Autodesk Inventor part; units mm, degrees
ref_plane "YZ Plane" through (0, 0, 0) normal (1, 0, 0) x (0, 1, 0)
ref_plane "XZ Plane" through (0, 0, 0) normal (0, 1, 0) x (-1, 0, 0)
ref_plane "XY Plane" through (0, 0, 0) normal (0, 0, 1) x (1, 0, 0)
sketch "Sketch1" plane through (0, 0, 0) normal (0, 1, 0) x (-1, 0, 0)
  line L0 (9, -10) -> (-9, -10)
  line L1 (-10, -9) -> (-10, 9)
  line L2 (-9, 10) -> (9, 10)
  line L3 (10, 9) -> (10, -9)
  line L4 (10, 10) -> (-10, -10) construction
  line L5 (10, -10) -> (-10, 10) construction
  arc A0 (10, 9) -> (9, 10) centre (9, 9) ccw
  arc A1 (9, -10) -> (10, -9) centre (9, -9) ccw
  arc A2 (-10, -9) -> (-9, -10) centre (-9, -9) ccw
  arc A3 (-9, 10) -> (-10, 9) centre (-9, 9) ccw
  point P0 (0, 0)
  point P1 (0, 0)
  dimension "d7" = 20
  dimension "d9" = 20
  dimension "d10" = 1
extrude "Extrusion1" add sketch "Sketch1" along normal blind 5
sketch "Sketch2" plane through (0, 5, 0) normal (0, 1, 0) x (1, 0, 0)
  line L0 (-10, 9) -> (-10, -9)
  arc A0 (-10, -9) -> (-9, -10) centre (-9, -9) ccw
  line L1 (-9, -10) -> (9, -10)
  arc A1 (9, -10) -> (10, -9) centre (9, -9) ccw
  line L2 (10, -9) -> (10, 9)
  arc A2 (10, 9) -> (9, 10) centre (9, 9) ccw
  line L3 (9, 10) -> (-9, 10)
  arc A3 (-9, 10) -> (-10, 9) centre (-9, 9) ccw
  line L4 (9, -11.5) -> (-9, -11.5)
  arc A4 (-11.5, -9) -> (-9, -11.5) centre (-9, -9) ccw
  line L5 (-11.5, -9) -> (-11.5, 9)
  arc A5 (-9, 11.5) -> (-11.5, 9) centre (-9, 9) ccw
  line L6 (-9, 11.5) -> (9, 11.5)
  arc A6 (11.5, 9) -> (9, 11.5) centre (9, 9) ccw
  line L7 (11.5, 9) -> (11.5, -9)
  arc A7 (9, -11.5) -> (11.5, -9) centre (9, -9) ccw
  circle A8 centre (0, 0) radius 2.75
  dimension "d16" = 1.5
  dimension "d19" = 5.5
extrude "Extrusion3" add sketch "Sketch2" along normal blind 1 contours A3 L3 A2 L2 A1 L1 A0 L0 | L4 A4 L5 A5 L6 A6 L7 A7
sketch "Sketch3" plane through (0, 0, 0) normal (0, -1, 0) x (1, 0, 0)
  circle A0 centre (0, 0) radius 4
  arc A1 (-6, -1) -> (-6, 1) centre (-6, 0) ccw
  arc A2 (-8, 1) -> (-8, -1) centre (-8, 0) ccw
  line L0 (-6, -1) -> (-8, -1)
  line L1 (-6, 1) -> (-8, 1)
  line L2 (0, 0) -> (-5, 0) construction
  arc A3 (-3.5355, -4.9497) -> (-4.9497, -3.5355) centre (-4.2426, -4.2426) ccw
  line L3 (-3.5355, -4.9497) -> (-4.9497, -6.364)
  line L4 (-4.9497, -3.5355) -> (-6.364, -4.9497)
  arc A4 (-6.364, -4.9497) -> (-4.9497, -6.364) centre (-5.6569, -5.6569) ccw
  arc A5 (1, -6) -> (-1, -6) centre (0, -6) ccw
  line L5 (1, -6) -> (1, -8)
  line L6 (-1, -6) -> (-1, -8)
  arc A6 (-1, -8) -> (1, -8) centre (0, -8) ccw
  arc A7 (4.9497, -3.5355) -> (3.5355, -4.9497) centre (4.2426, -4.2426) ccw
  line L7 (4.9497, -3.5355) -> (6.364, -4.9497)
  line L8 (3.5355, -4.9497) -> (4.9497, -6.364)
  arc A8 (4.9497, -6.364) -> (6.364, -4.9497) centre (5.6569, -5.6569) ccw
  arc A9 (6, 1) -> (6, -1) centre (6, 0) ccw
  line L9 (6, 1) -> (8, 1)
  line L10 (6, -1) -> (8, -1)
  arc A10 (8, -1) -> (8, 1) centre (8, 0) ccw
  arc A11 (3.5355, 4.9497) -> (4.9497, 3.5355) centre (4.2426, 4.2426) ccw
  line L11 (3.5355, 4.9497) -> (4.9497, 6.364)
  line L12 (4.9497, 3.5355) -> (6.364, 4.9497)
  arc A12 (6.364, 4.9497) -> (4.9497, 6.364) centre (5.6569, 5.6569) ccw
  arc A13 (-1, 6) -> (1, 6) centre (0, 6) ccw
  line L13 (-1, 6) -> (-1, 8)
  line L14 (1, 6) -> (1, 8)
  arc A14 (1, 8) -> (-1, 8) centre (0, 8) ccw
  arc A15 (-4.9497, 3.5355) -> (-3.5355, 4.9497) centre (-4.2426, 4.2426) ccw
  line L15 (-4.9497, 3.5355) -> (-6.364, 4.9497)
  line L16 (-3.5355, 4.9497) -> (-4.9497, 6.364)
  arc A16 (-4.9497, 6.364) -> (-6.364, 4.9497) centre (-5.6569, 5.6569) ccw
  dimension "d24" = 2
  dimension "d25" = 2
  dimension "d26" = 2
  dimension "d27" = 6
  dimension "d28" = 360
  dimension "d29" = 16
  dimension "d37" = 8
extrude "Extrusion4" cut sketch "Sketch3" against normal blind 1
hole "Hole1" at (0, 5, 0) direction (0, -1, 0) diameter 5.5 depth 3
equation "\"d7\" = button_side"
equation "\"d9\" = d7"
equation "\"d24\" = d25"
equation "\"d25\" = d26"
equation "\"d37\" = 4 * d26"
equation "\"d0\" = 122"
equation "\"d1\" = 77"
equation "\"d4\" = 19"
equation "\"d5\" = 1"
equation "\"d8\" = 25"
equation "\"d13\" = 1.5"
equation "\"d14\" = 0"
equation "\"d15\" = 2"
equation "\"d30\" = 3.1"
equation "\"d31\" = 3"
equation "\"d33\" = 3"
equation "\"d34\" = 2"
equation "\"d36\" = 3"
equation "\"d38\" = 90deg"
equation "\"d39\" = 8"
equation "\"d40\" = 118deg"
equation "\"d44\" = 0"
equation "\"d45\" = 1.2"
equation "\"d46\" = 2"
equation "\"d47\" = 0"
equation "\"d50\" = 25"
equation "\"button_side\" = 20"
equation "\"d3\" = 1.01 * button_side"
equation "\"d2\" = d3"
properties part number "button1" material "Bronze, Soft Tin"
Verification items for the finished model (mm, model axes). A direction names the side the tool comes from. Coordinates: 2 decimals unless noted, no trailing zeros. Write each loop counter-clockwise with the first axis right and the second up, starting at its lowest first coordinate (ties: lowest second). Pieces come first, ordered by that corner, then holes. Notation, with made-up numbers: M -25.5,-21.75 L 8.5,-21.75 A21 ccw 8.5,-9.75 Z; hole C -17,87.25 d1. An arc over 180 degrees is marked long. One line per question, with ' | ' between items.
1) Sectioned sample at C-C on x = -2.25. Record the cut outline in (y, z), then the cut area to 3 significant figures.
Solutions:
outline: M 0,-10 L 5,-10 L 5,-11.5 L 6,-11.5 L 6,-1.58 L 2,-1.58 L 2,1.58 L 6,1.58 L 6,11.5 L 5,11.5 L 5,10 L 0,10 L 0,3.31 L 1,3.31 L 1,-3.31 L 0,-3.31 Z | area: 104 mm^2
2) Sectioned sample at A-A on y = 4.1. Record the cut outline in (x, z).
Solutions:
outline: M -10,-9 A1 ccw -9,-10 L 9,-10 A1 ccw 10,-9 L 10,9 A1 ccw 9,10 L -9,10 A1 ccw -10,9 Z; hole C 0,0 d5.5
3) Release check for a two-part mould opening along Z. For faces 1 (the face through (-9.699, 2.465, 9.715)), 2 (the face through (-11.5, 5.5, 0.1)), 3 (the face through (-0.1, 5.5, -11.5)), 4 (the face through (0, 0.5, -9)) record: +Z half, -Z half, draft (parallel to the pull), parting line (faces both ways), or undercut.
Solutions:
face 1: +Z half | face 2: draft | face 3: -Z half | face 4: undercut
4) Sectioned sample at B-B on y = 1.3. Record the cut outline in (x, z).
Solutions:
outline: M -10,-9 A1 ccw -9,-10 L 9,-10 A1 ccw 10,-9 L 10,9 A1 ccw 9,10 L -9,10 A1 ccw -10,9 Z
5) Depth check by flat-ended pin: pin 1 Ø2.5 at (x, y) = (-0.5, 3) entering from +Z; pin 2 Ø1 at (y, z) = (2, -8) entering from -X; pin 3 Ø1.1 at (x, y) = (-7, 0.5) entering from -Z. Enter the tip coordinate at first touch or a pass-through.
Solutions:
pin 1: z = 10 | pin 2: x = -10 | pin 3: z = -10
6) Material ranges on L1, parallel to Z at x = 0, y = 0.45; L2, parallel to Z at x = 0, y = 3.3; L3, parallel to Z at x = 3.5, y = 0.6, recorded low to high.
Solutions:
L1: -10 to -9, -5 to -4, 4 to 5, 9 to 10 | L2: -10 to -2.75, 2.75 to 10 | L3: -10 to -4.91, -3.57 to -1.94, 1.94 to 3.57, 4.91 to 10
7) Access from +Z, -Z, +X, -X, +Y, -Y to the whole of each face (thin tool, end or side, straight path). Record for faces 5 (the face through (3.52, 0.49, 3.55)), 6 (the face through (-10, 2, 0)), 7 (the face through (-3, 6, -3)), 8 (the face through (-9.715, 2.465, -9.699)), 9 (the face through (0, 2, -10)).
Solutions:
face 5: -Y | face 6: +Z, -Z, -X, -Y | face 7: +Z, -Z, +X, -X, +Y | face 8: -Z, -X, -Y | face 9: -Z, +X, -X, -Y
